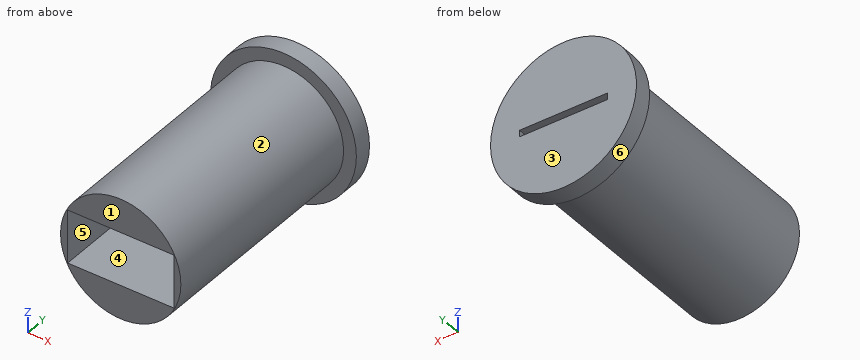
Autodesk Fusion 360 part; units mm, degrees
sketch "Esquisse1" plane through (0, 0, 0) normal (0, 1, 0) x (1, 0, 0)
  circle A0 centre (0, 0) radius 20
  circle A1 centre (0, 0) radius 16.5
  line L0 (12.05, 0.9) -> (-12.05, 0.9)
  line L1 (-12.05, 0.9) -> (-12.05, -0.9)
  line L2 (-12.05, -0.9) -> (12.05, -0.9)
  line L3 (12.05, -0.9) -> (12.05, 0.9)
  line L4 (12.05, 0.9) -> (-12.05, -0.9) construction
  line L5 (-12.05, 0.9) -> (12.05, -0.9) construction
  line L6 (14.55, -7.3) -> (-14.55, -7.3)
  line L7 (-14.55, -7.3) -> (-14.55, 7.3)
  line L8 (-14.55, 7.3) -> (14.55, 7.3)
  line L9 (14.55, 7.3) -> (14.55, -7.3)
  line L10 (14.55, -7.3) -> (-14.55, 7.3) construction
  line L11 (-14.55, -7.3) -> (14.55, 7.3) construction
  dimension "d1" = 40
  dimension "d2" = 33
  dimension "d3" = 24.1
  dimension "d4" = 1.8
  dimension "d6" = 29.1
  dimension "d7" = 14.6
extrude "Extrusion1" add sketch "Esquisse1" along normal blind 5 contours A0 | A1 | L6 L7 L8 L9
extrude "Extrusion2" add sketch "Esquisse1" against normal blind 12 contours A1 | L6 L7 L8 L9
extrude "Extrusion3" add sketch "Esquisse1" against normal blind 62 contours A1
equation "d3 = 23.9 mm + err"
equation "d4 = 1.6 mm + ( err )"
equation "err = erreur de l'impression"
equation "d6 = 28.9 mm + err"
equation "d7 = 14.4 mm + err"
equation "d12 = -12 mm - 50 mm"
Here's how the part is built. I have some questions about the finished solid (model axes, mm). Face numbers are marked on the shaded views. A direction names the side the tool comes from. Coordinates: 2 decimals unless noted, no trailing zeros. Loops run counter-clockwise (first coordinate to the right, second up) from the corner with the lowest first, then second, coordinate; pieces in that order, holes last. Notation, with made-up numbers: M 88,79.25 L 121,79.25 A29 cw 121,118.25 Z; hole C -20,-20 d6. An arc over 180 degrees is marked long. One line per item, written item: value.
1. Imagine slicing it at D-D (x = 13). List the corners of the cut face in (y, z) for me, and give its area (3 significant figures).
Geometry says:
outline: M -62,-10.16 L 0,-10.16 L 0,-15.2 L 5,-15.2 L 5,15.2 L 0,15.2 L 0,10.16 L -62,10.16 L -62,7.3 L -12,7.3 L -12,-7.3 L -62,-7.3 Z
area: 682 mm2
2. Imagine slicing it at C-C (y = -58). List the corners of the cut face in (x, z) for me.
Geometry says:
outline: C 0,0 d33; hole M -14.55,-7.3 L 14.55,-7.3 L 14.55,7.3 L -14.55,7.3 Z
3. Will these pins go through, and if not, where does the flat tip stop? pin 1 Ø2 at (y, z) = (-52.5, 7) entering from -X; pin 2 Ø1.4 at (y, z) = (-4.5, 0) entering from -X; pin 3 Ø8 at (x, y) = (4, -27.5) entering from -Z.
Geometry says:
pin 1: stops at x = -15.37
pin 2: stops at x = -16.5
pin 3: stops at z = -16.5
4. Imagine slicing it at B-B (x = 0). List the corners of the cut face in (y, z) for me.
Geometry says:
outline: M -62,-16.5 L 0,-16.5 L 0,-20 L 5,-20 L 5,-0.9 L -12,-0.9 L -12,-7.3 L -62,-7.3 Z; M -62,7.3 L -12,7.3 L -12,0.9 L 5,0.9 L 5,20 L 0,20 L 0,16.5 L -62,16.5 Z
5. Thinking about a two-plate mould opening in Z: for the marked faces 3, 4, 5 and 6, which applies, +Z half, -Z half, draft (parallel to the pull), parting line (faces both ways), or undercut?
Geometry says:
face 3: draft
face 4: undercut
face 5: undercut
face 6: parting line
6. Imagine slicing it at A-A (z = 0). List the corners of the cut face in (x, y) for me, and give its area (3 significant figures).
Geometry says:
outline: M -20,0 L -16.5,0 L -16.5,-62 L -14.55,-62 L -14.55,-12 L -12.05,-12 L -12.05,5 L -20,5 Z; M 12.05,-12 L 14.55,-12 L 14.55,-62 L 16.5,-62 L 16.5,0 L 20,0 L 20,5 L 12.05,5 Z
area: 381 mm2
7. On a 3-axis mill with a long thin cutter (end or side, diameter ignored), from which of +Z, -Z, +X, -X, +Y, -Y can I reach the whole of each face in a straight line? I mean the marked faces 1 and 2. Say none if no direction works.
Geometry says:
face 1: +Z, -Z, +X, -X, -Y
face 2: -Y
8. Please list where these lines run through material, in increasing order: probe 1 along Z at (x, y) = (3.5, -51.5); probe 2 along Z at (x, y) = (5, -40.5); probe 3 along X at (y, z) = (-16.5, 1).
Geometry says:
probe 1: z = -16.12 to -7.3, 7.3 to 16.12
probe 2: z = -15.72 to -7.3, 7.3 to 15.72
probe 3: x = -16.47 to -14.55, 14.55 to 16.47
